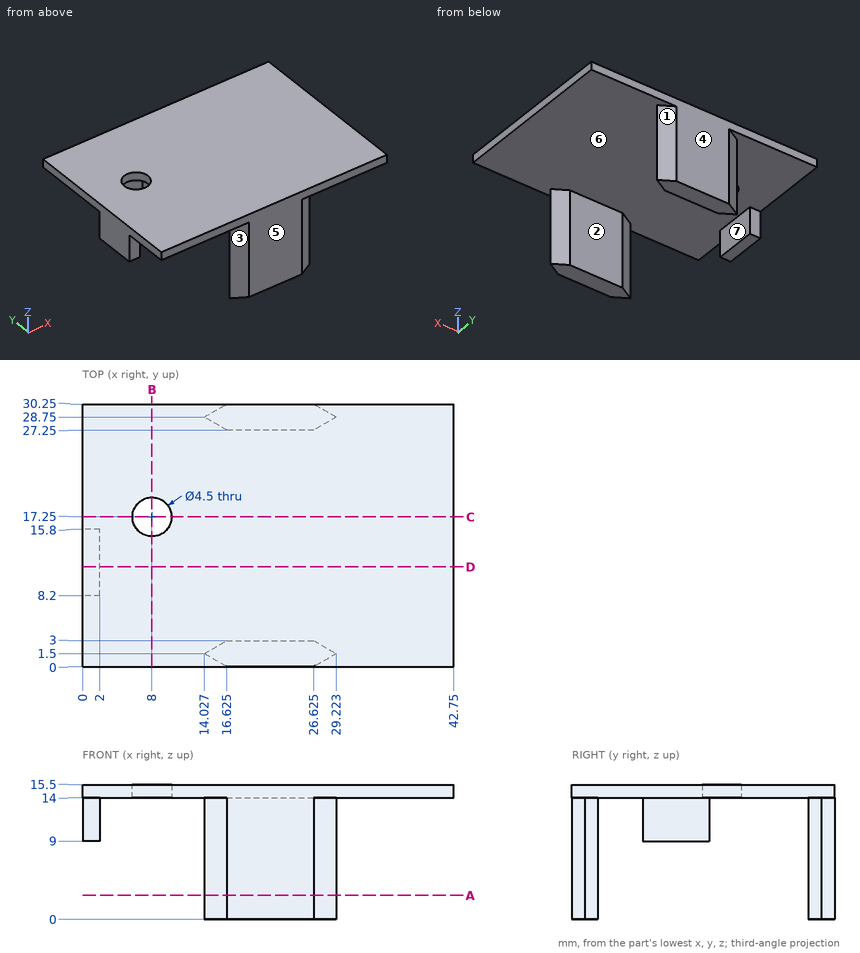
Source: three-view drawing plus pictorial views. Frame: mm from the lowest corner of the part. A direction names the side the tool comes from. Round coordinates to 2 decimals unless told otherwise and drop trailing zeros. Loops run counter-clockwise (first coordinate to the right, second up) from the corner with the lowest first, then second, coordinate; pieces in that order, holes last. Notation, with made-up numbers: (46, 81) - (97, 81) arc R25 ccw to (97, 116) - close; hole circle Ø7 at (-5, -19.75). An arc over 180 degrees is marked (long way). Write each question's results on one line, items separated by ' | '. Start each with the question number.
1) Cut plane D-D on y = 11.5. Return loops of the section in (x, z), then the cut area to 3 significant figures.
2) First-contact query: P1, Ø2, axis at x = 1, z = 12.5, coming from the +Y side; P2, Ø1, axis at x = 1.5, z = 12, coming from the -Y side; P3, Ø0.6, axis at x = 1.5, y = 12.5, coming from the -Z side. Flat tips, straight axial feed; report the tip coordinate or a pass-through.
3) Cut plane C-C on y = 17.25. Return loops of the section in (x, z).
4) Line query: probe 1 along Y at (x, z) = (8, 14.8); probe 2 along Z at (x, y) = (33, 1.5); probe 3 along Y at (x, z) = (23.5, 8.5). Output: solid intervals per line, ascending. Write a range as [from, to].
5) Cut plane B-B on x = 8. Return loops of the section in (y, z).
6) Access query for the marked faces 1, 2 and 3. Directions: +Z, -Z, +X, -X, +Y, -Y. A direction counts if a zero-diameter tool reaches every point of the face in a straight line with its end or side. Return the directions, or none.
7) Mould query, pull axis Y, two halves, no side actions, for the marked faces 4, 5, 6 and 7. Classes: released by +Y, released by -Y, zero draft, split by the parting line, or undercut.
8) Cut plane A-A on z = 2.75. Return loops of the section in (x, y) (3 decimals).
Verdict:
1) outline: (0, 9) - (2, 9) - (2, 14) - (42.75, 14) - (42.75, 15.5) - (0, 15.5) - close | area: 74.1 mm2
2) P1: stops at y = 15.8 | P2: stops at y = 8.2 | P3: stops at z = 9
3) outline: (0, 14) - (5.75, 14) - (5.75, 15.5) - (0, 15.5) - close; (10.25, 14) - (42.75, 14) - (42.75, 15.5) - (10.25, 15.5) - close
4) probe 1: y = [0, 15], [19.5, 30.25] | probe 2: z = [14, 15.5] | probe 3: y = [0, 3], [27.25, 30.25]
5) outline: (0, 14) - (15, 14) - (15, 15.5) - (0, 15.5) - close; (19.5, 14) - (30.25, 14) - (30.25, 15.5) - (19.5, 15.5) - close
6) face 1: -Z, +X, +Y | face 2: -Z, +X, -X | face 3: -Z, -X, -Y
7) face 4: released by +Y | face 5: released by -Y | face 6: undercut | face 7: zero draft
8) outline: (14.027, 1.5) - (16.625, 0) - (26.625, 0) - (29.223, 1.5) - (26.625, 3) - (16.625, 3) - close; (14.027, 28.75) - (16.625, 27.25) - (26.625, 27.25) - (29.223, 28.75) - (26.625, 30.25) - (16.625, 30.25) - close
